from build123d import *

# Parameters (mm, degrees)
SKETCH_1_R      = 1.1
EXTRUDE_1_DEPTH = 13
FILLET_1_R      = 1


with BuildPart() as part:
    # 草图1 → 凸台-拉伸1 (new body)
    with BuildSketch(Plane(origin=(0, 0, 0), x_dir=(0, 0, -1), z_dir=(1, 0, 0))):
        Polygon((3.25, 7), (-3.25, 7), (-3.25, 1), (1.95, 1), (1.95, -1), (-3.25, -1), (-3.25, -7), (3.25, -7), align=None)
        with Locations((0, -4)):
            Circle(SKETCH_1_R, mode=Mode.SUBTRACT)
        with Locations((0, 4)):
            Circle(SKETCH_1_R, mode=Mode.SUBTRACT)
    extrude(amount=-EXTRUDE_1_DEPTH)

    # 圆角1
    fillet_1_edges = [part.edges().sort_by_distance(p)[0] for p in [
        (-6.5, 1, 3.25),
        (-6.5, 7, 3.25),
        (-6.5, 7, -3.25),
        (-6.5, -7, -3.25),
        (-6.5, -7, 3.25),
        (-6.5, -1, 3.25),
    ]]
    fillet(fillet_1_edges, radius=FILLET_1_R)


solid = part.part
The model under review builds one solid part; all positions refer to its coordinate system, in mm. A direction names the side the tool comes from. Give positions to 0.01 mm unless a question says otherwise; leave off trailing zeros. Loops run counter-clockwise (first coordinate to the right, second up) from the corner with the lowest first, then second, coordinate; pieces in that order, holes last. Notation, with made-up numbers: (80, 45) -> (87, 45) arc R10 cw to (87, 61) -> close; hole circle Ø8 at (46, -26). An arc over 180 degrees is marked (long way). Put each result on its own line as item: value. Start each with the question number.
1. We need section D-D on z = 2.5. State the section outline as (x, y) points, then the cut area to 3 significant figures.
2. We need section C-C on x = -2.75. State the section outline as (y, z) points.
3. For faces 4 (the face through (-6.591, 1.301, 2.965)), 5 (the face through (-6.591, -6.715, 2.949)), list the 3-axis set-ups (+Z, -Z, +X, -X, +Y, -Y) from which the entire face can be reached by the end or side of a thin tool; tool diameter is ignored.
4. We need section B-B on y = 4. State the section outline as (x, z) points.
5. We need section A-A on z = 0. State the section outline as (x, y) points.
6. Clearance check with flat-ended pins moving along their axes: P1, Ø0.6, axis at x = -9.5, y = 0.5, coming from the +Z side; P2, Ø2, axis at y = -4, z = 0, coming from the -X side. State where each tip first meets the part, or that it passes through.
7. Mouldability with a two-part tool opening along Y and no side actions: class faces 1 (the face through (-6, 0, -3.25)), 2 (the face through (-6, -1, 0)), 3 (the face through (-6.591, 6.715, 2.949)) as released by +Y, released by -Y, zero draft, split by the parting line, or undercut.
8. Wall thickness on probe 1 along Y at (x, z) = (-4, 0); probe 2 along Y at (x, z) = (-4, 1.5); probe 3 along Y at (x, z) = (-6.5, 0.5): over which ranges is each line inside the solid? List them lowest first.
Determined:
1. outline: (-13, -6.97) -> (0, -6.97) -> (0, -1.03) -> (-13, -1.03) -> close; (-13, 1.03) -> (0, 1.03) -> (0, 6.97) -> (-13, 6.97) -> close
1. area: 154 mm^2
2. outline: (-7, -2.25) arc R1 ccw to (-6, -3.25) -> (6, -3.25) arc R1 ccw to (7, -2.25) -> (7, 2.25) arc R1 ccw to (6, 3.25) -> (2, 3.25) arc R1 ccw to (1, 2.25) -> (1, -1.95) -> (-1, -1.95) -> (-1, 2.25) arc R1 ccw to (-2, 3.25) -> (-6, 3.25) arc R1 ccw to (-7, 2.25) -> close; hole circle Ø2.2 at (-4, 0); hole circle Ø2.2 at (4, 0)
3. face 4: +Z, +X, -X
3. face 5: +Z, +X, -X, -Y
4. outline: (-13, -3.25) -> (0, -3.25) -> (0, -1.1) -> (-13, -1.1) -> close; (-13, 1.1) -> (0, 1.1) -> (0, 3.25) -> (-13, 3.25) -> close
5. outline: (-13, -7) -> (0, -7) -> (0, -5.1) -> (-13, -5.1) -> close; (-13, -2.9) -> (0, -2.9) -> (0, -1) -> (-13, -1) -> close; (-13, 1) -> (0, 1) -> (0, 2.9) -> (-13, 2.9) -> close; (-13, 5.1) -> (0, 5.1) -> (0, 7) -> (-13, 7) -> close
6. P1: z = -1.95
6. P2: through
7. face 1: zero draft
7. face 2: undercut
7. face 3: released by +Y
8. probe 1: -7 to -5.1, -2.9 to -1, 1 to 2.9, 5.1 to 7
8. probe 2: -7 to -1, 1 to 7
8. probe 3: -7 to -4.98, -3.02 to -1, 1 to 3.02, 4.98 to 7
